Source: CAD feature listing. Evaluate the final solid. Frame: model axes, mm. Round coordinates to 2 decimals unless told otherwise and drop trailing zeros. Write each loop counter-clockwise with the first axis right and the second up, starting at its lowest first coordinate (ties: lowest second). Pieces come first, ordered by that corner, then holes. Notation, with made-up numbers: M -32.5,30 L -23.5,30 A25 ccw -23.5,62 Z; hole C -39.75,34 d8. An arc over 180 degrees is marked long. Answer in a Markdown table with one row per item. Add a question column.
Item 1: Contact query for a flat-ended pin moving along its axis: pin 1 (1.5 mm diameter, centred on y = 27, z = -2.5, fed in from +X). Output: stop coordinate, or through.
Item 2: Cut plane A-A on y = 34.5. Return loops of the section in (x, z) (1 decimal), and give its area (3 significant figures).
Item 3: Material intervals for probe 1 along Y at (x, z) = (2.5, -1.75); probe 2 along X at (y, z) = (46, -1.75); probe 3 along X at (y, z) = (63, 2.5), sorted ascending.
Autodesk Inventor part; units mm, degrees
ref_plane "YZ Plane" through (0, 0, 0) normal (1, 0, 0) x (0, 1, 0)
ref_plane "XZ Plane" through (0, 0, 0) normal (0, 1, 0) x (-1, 0, 0)
ref_plane "XY Plane" through (0, 0, 0) normal (0, 0, 1) x (1, 0, 0)
sketch "Sketch1" plane through (0, 0, 0) normal (0, 1, 0) x (-1, 0, 0)
  line L0 (-3.175, -3.175) -> (3.175, -3.175)
  line L1 (3.175, -3.175) -> (3.175, 3.175)
  line L2 (3.175, 3.175) -> (-3.175, 3.175)
  line L3 (-3.175, 3.175) -> (-3.175, -3.175)
  line L4 (-3.175, -3.175) -> (3.175, 3.175) construction
  line L5 (3.175, -3.175) -> (-3.175, 3.175) construction
  point P0 (0, 0)
  dimension "d2" = 6.35
  dimension "d3" = 6.35
extrude "Extrusion1" add sketch "Sketch1" along normal blind 91.44
fillet "Fillet1" radius 1.5875 4 edges at (3.175, 45.72, 3.175) (3.175, 45.72, -3.175) (-3.175, 45.72, -3.175) (-3.175, 45.72, 3.175)
fillet "Fillet2" radius 0.7937 16 edges at (3.175, 0, 0) (2.71, 0, -2.71) (0, 0, -3.175) (-2.71, 0, -2.71) (-3.175, 0, 0) (-2.71, 0, 2.71) (0, 0, 3.175) (2.71, 0, 2.71) (0, 91.44, 3.175) (-2.71, 91.44, 2.71) (-3.175, 91.44, 0) (-2.71, 91.44, -2.71) (0, 91.44, -3.175) (2.71, 91.44, -2.71) (3.175, 91.44, 0) (2.71, 91.44, 2.71)
properties part number "wedgea" material "Stainless Steel"
Results below:
| question | item | result |
|---|---|---|
| 1 | pin 1 | x = 3.17 |
| 2 | outline | M -3.2,-1.6 A1.6 ccw -1.6,-3.2 L 1.6,-3.2 A1.6 ccw 3.2,-1.6 L 3.2,1.6 A1.6 ccw 1.6,3.2 L -1.6,3.2 A1.6 ccw -3.2,1.6 Z |
| 2 | area | 38.2 mm2 |
| 3 | probe 1 | 0.01 to 91.43 |
| 3 | probe 2 | -3.17 to 3.17 |
| 3 | probe 3 | -2.89 to 2.89 |
